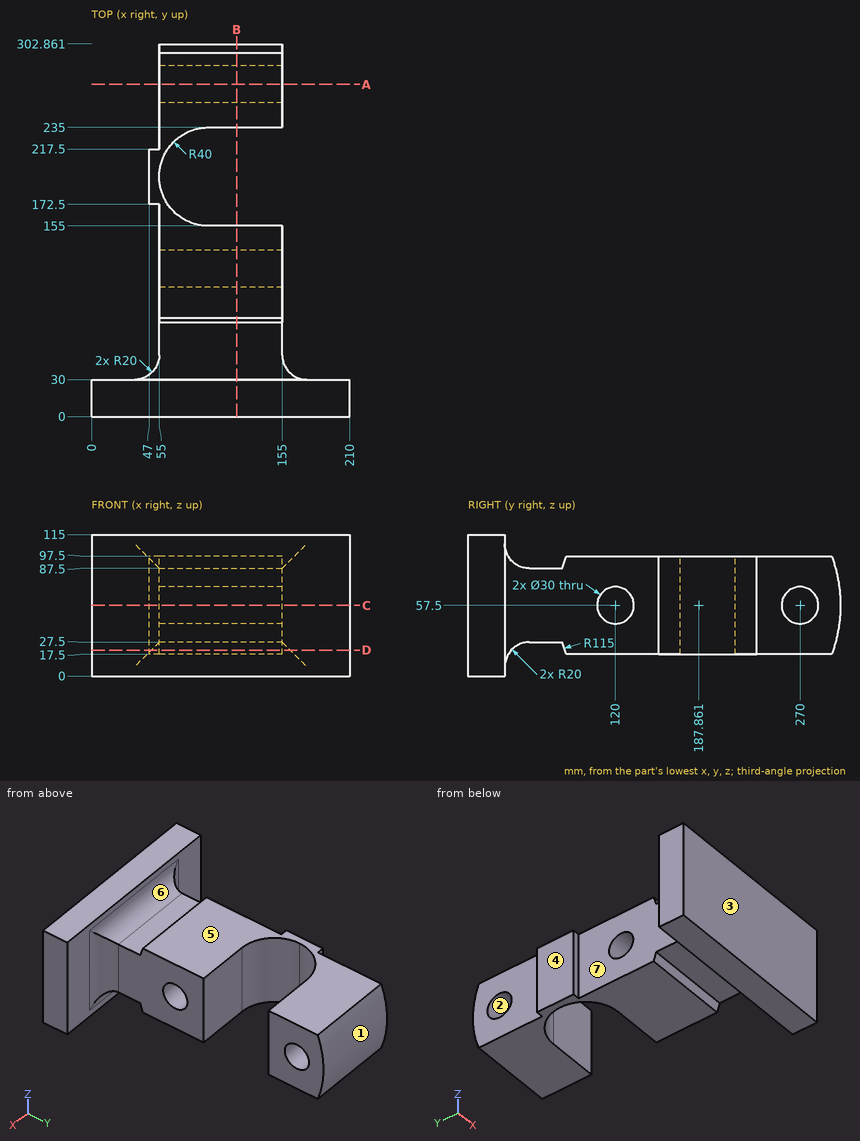
Geometry: see drawing. Coordinates: mm, zero at the bounding-box minimum. A direction names the side the tool comes from. Coordinates: 2 decimals unless noted, no trailing zeros. Write each loop counter-clockwise with the first axis right and the second up, starting at its lowest first coordinate (ties: lowest second). Pieces come first, ordered by that corner, then holes.
1) Pin query (flat end, axial travel): pin 1 Ø1.5 at (y, z) = (63, 65) entering from -X; pin 2 Ø1 at (x, z) = (107.5, 61) entering from -Y; pin 3 Ø10 at (y, z) = (74, 94) entering from +X; pin 4 Ø2.5 at (x, z) = (50.5, 68) entering from +Y. Return the tip coordinate at first contact, or that it passes through.
2) Material intervals for line 1 along Y through (x, z) = (103, 57); line 2 along X through (y, z) = (237.5, 78.5); line 3 along Y through (x, z) = (201, 21), sorted ascending.
3) Section A-A on y = 270. Output: boundary loops of the cut face in (x, z), and give its area (3 significant figures).
4) Section B-B on x = 118. Output: boundary loops of the cut face in (y, z), and give its area (3 significant figures).
5) Mould query, pull axis Z, two halves, no side actions, for the marked faces 1, 2 and 3. Classes: pulls with the +Z half, pulls with the -Z half, needs draft (parallel to the pull), parting line crosses it, or undercut.
6) Section C-C on z = 57.5. Output: boundary loops of the cut face in (x, y), and give its area (3 significant figures).
7) Set-up query: the marked faces 4, 5, 6 and 7. Return all of +Z, -Z, +X, -X, +Y, -Y with unobstructed straight access to the full face (end or side cutting, diameter ignored); none if empty.
8) Section D-D on z = 21. Output: boundary loops of the cut face in (x, y) (1 decimal).
Check result:
1. pin 1: stops at x = 55
1. pin 2: stops at y = 0
1. pin 3: stops at x = 155
1. pin 4: stops at y = 217.5
2. line 1: y = 0 to 105.01, 134.99 to 155, 235 to 255.01, 284.99 to 302.86
2. line 2: x = 55 to 155
2. line 3: y = 0 to 30
3. outline: (55, 17.5) - (155, 17.5) - (155, 42.5) - (55, 42.5) - close; (55, 72.5) - (155, 72.5) - (155, 97.5) - (55, 97.5) - close
3. area: 5,000 mm2
4. outline: (0, 0) - (30, 0) - (30, 7.5) arc R20 cw to (50, 27.5) - (76.84, 27.5) arc R115 ccw to (80.04, 17.5) - (155, 17.5) - (155, 97.5) - (80.04, 97.5) arc R115 ccw to (76.84, 87.5) - (50, 87.5) arc R20 cw to (30, 107.5) - (30, 115) - (0, 115) - close; (235, 17.5) - (295.68, 17.5) arc R115 ccw to (295.68, 97.5) - (235, 97.5) - close; hole circle Ø30 at (120, 57.5); hole circle Ø30 at (270, 57.5)
4. area: 16,500 mm2
5. face 1: parting line crosses it
5. face 2: undercut
5. face 3: needs draft
6. outline: (0, 0) - (210, 0) - (210, 30) - (175, 30) arc R20 cw to (155, 50) - (155, 105) - (55, 105) - (55, 50) arc R20 cw to (35, 30) - (0, 30) - close; (47, 172.5) - (55, 172.5) - (55, 135) - (155, 135) - (155, 155) - (95, 155) arc R40 cw to (95, 235) - (155, 235) - (155, 255) - (55, 255) - (55, 217.5) - (47, 217.5) - close; (55, 285) - (155, 285) - (155, 302.86) - (55, 302.86) - close
6. area: 20,800 mm2
7. face 4: +Z, -Z, -X, +Y
7. face 5: +Z, +X, -X, +Y
7. face 6: +Z, +X, -X
7. face 7: +Z, -Z, -X
8. outline: (0, 0) - (210, 0) - (210, 30) - (175, 30) arc R20 cw to (161.5, 35.2) - (48.5, 35.2) arc R20 cw to (35, 30) - (0, 30) - close; (47, 172.5) - (55, 172.5) - (55, 78.8) - (155, 78.8) - (155, 155) - (95, 155) arc R40 cw to (95, 235) - (155, 235) - (155, 296.9) - (55, 296.9) - (55, 217.5) - (47, 217.5) - close
